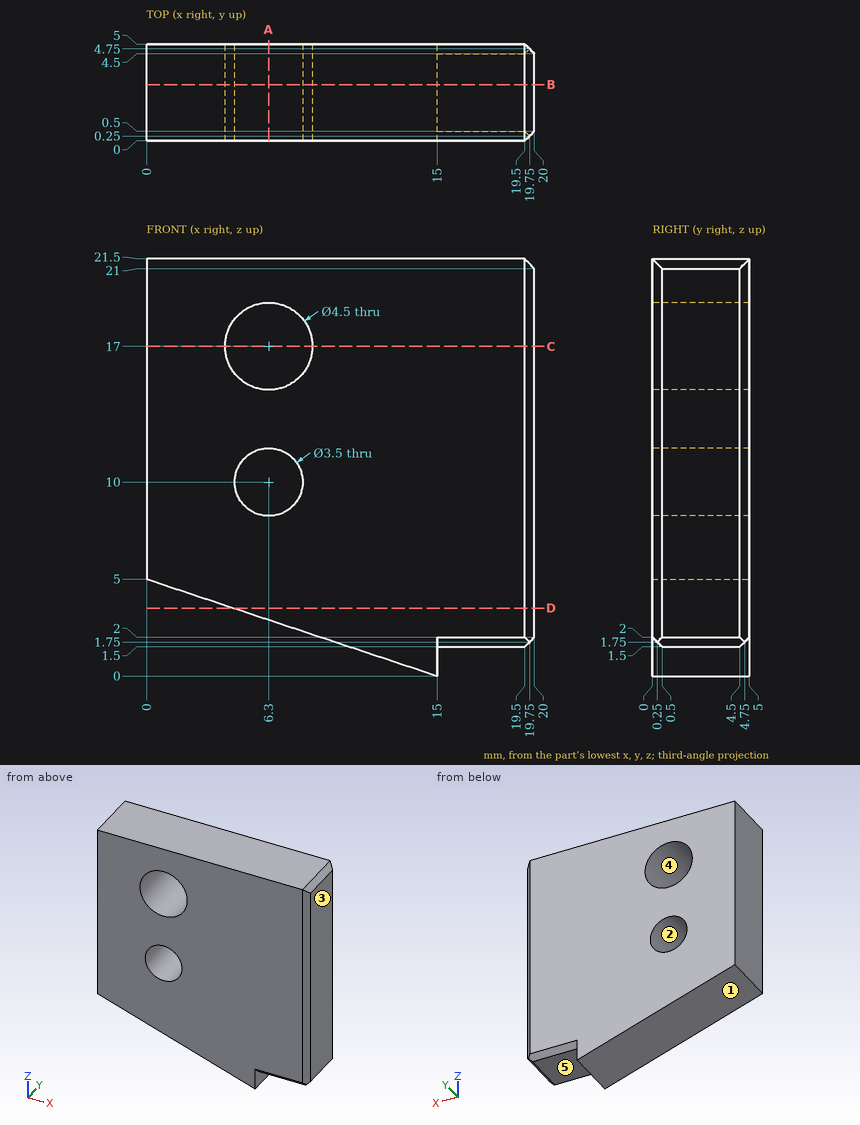
Can you work these out from the drawing? Everything is in mm from the part's minimum corner. A direction names the side the tool comes from. Round coordinates to 2 decimals unless told otherwise and drop trailing zeros. Write each loop counter-clockwise with the first axis right and the second up, starting at its lowest first coordinate (ties: lowest second). Pieces come first, ordered by that corner, then holes.
1. For the marked faces 4 and 5, which set-ups out of +Z, -Z, +X, -X, +Y, -Y let a thin tool reach every point of the face, with its end or its side?
2. Suppose I cut it at B-B (y = 2.9). List the corners of the cut face in (x, z) for me, and give its area (3 significant figures).
3. Suppose I cut it at A-A (x = 6.3). List the corners of the cut face in (y, z) for me.
4. I need wall thicknesses on L1, parallel to Z at x = 6.3, y = 2.05; L2, parallel to Z at x = 5, y = 4.25; L3, parallel to Z at x = 17.5, y = 3.7. Which ranges of each line are inside material? Lowest first, please.
5. Suppose I cut it at C-C (z = 17). List the corners of the cut face in (x, y) for me, and give its area (4 significant figures).
6. If we mould it in two halves opening along Z, with no side actions, what happens to the marked faces 1, 2 and 3? For each: released by +Z, released by -Z, zero draft, split by the parting line, or undercut.
7. Suppose I cut it at D-D (z = 3.5). List the corners of the cut face in (x, y) for me, and give its area (4 significant figures).
8. Will these pins go through, and if not, where does the flat tip stop? pin 1 Ø3 at (x, y) = (4, 1.5) entering from -Z; pin 2 Ø1.5 at (x, y) = (4.5, 2.5) entering from -Z.
Answer sheet:
1. face 4: +Y, -Y
1. face 5: -Z, +X, +Y, -Y
2. outline: (0, 5) - (15, 0) - (15, 1.5) - (19.5, 1.5) - (20, 2) - (20, 21) - (19.5, 21.5) - (0, 21.5) - close; hole circle Ø4.5 at (6.3, 17); hole circle Ø3.5 at (6.3, 10)
2. area: 359 mm2
3. outline: (0, 2.9) - (5, 2.9) - (5, 8.25) - (0, 8.25) - close; (0, 11.75) - (5, 11.75) - (5, 14.75) - (0, 14.75) - close; (0, 19.25) - (5, 19.25) - (5, 21.5) - (0, 21.5) - close
4. L1: z = 2.9 to 8.25, 11.75 to 14.75, 19.25 to 21.5
4. L2: z = 3.33 to 8.83, 11.17 to 15.16, 18.84 to 21.5
4. L3: z = 1.5 to 21.5
5. outline: (0, 0) - (4.05, 0) - (4.05, 5) - (0, 5) - close; (8.55, 0) - (19.5, 0) - (20, 0.5) - (20, 4.5) - (19.5, 5) - (8.55, 5) - close
5. area: 77.25 mm2
6. face 1: released by -Z
6. face 2: undercut
6. face 3: zero draft
7. outline: (4.5, 0) - (19.5, 0) - (20, 0.5) - (20, 4.5) - (19.5, 5) - (4.5, 5) - close
7. area: 77.25 mm2
8. pin 1: stops at z = 3.17
8. pin 2: stops at z = 3.25
